Source: CAD feature listing. Evaluate the final solid. Frame: model axes, mm. Round coordinates to 2 decimals unless told otherwise and drop trailing zeros. Loops run counter-clockwise (first coordinate to the right, second up) from the corner with the lowest first, then second, coordinate; pieces in that order, holes last. Notation, with made-up numbers: (-5, 17) -> (28, 17) arc R24 cw to (28, 30) -> close; hole circle Ø3 at (20, 25.5). An arc over 180 degrees is marked (long way). Write item = value, one per line.
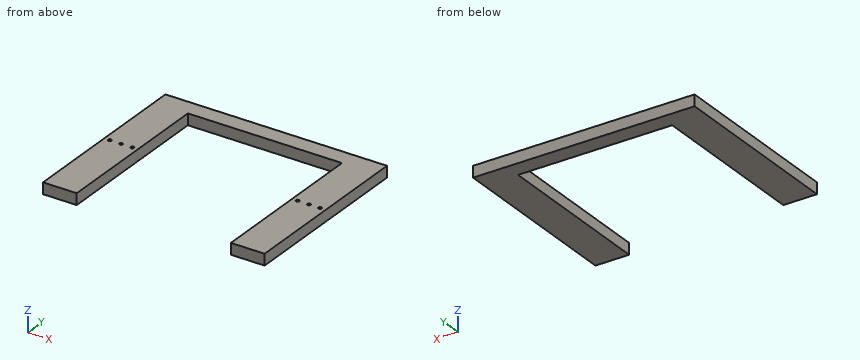
from build123d import *

# Parameters (mm, degrees)
SKETCH_1_W          = 60
SKETCH_1_H          = 325
EXTRUDE_1_DEPTH     = 20
EXTRUDE_1_2_DEPTH   = 20
SKETCH_3_R          = 3
CUT_EXTRUDE_1_DEPTH = 10
SKETCH_5_W          = 274
SKETCH_5_H          = 30
EXTRUDE_2_DEPTH     = 20


with BuildPart() as part:
    # Sketch 1 → Extrude 1 (new body)
    with BuildSketch(Plane.XY):
        with Locations((30, -162.5)):
            Rectangle(SKETCH_1_W, SKETCH_1_H)
    extrude(amount=EXTRUDE_1_DEPTH)


with BuildPart() as body_2:
    # Sketch 1 → Extrude 1 2 (new body)
    with BuildSketch(Plane.XY):
        with Locations((-304, -162.5)):
            Rectangle(SKETCH_1_W, SKETCH_1_H)
    extrude(amount=EXTRUDE_1_2_DEPTH)


with BuildPart() as cut_extrude_1_tool:
    # Sketch 3 → Cut-Extrude 1 (new body)
    with BuildSketch(Plane.XY.offset(20)):
        with Locations((50, -162.5)):
            Circle(SKETCH_3_R)
        with Locations((10, -162.5)):
            Circle(SKETCH_3_R)
        with Locations((30, -162.5)):
            Circle(SKETCH_3_R)
        with Locations((-324, -162.5)):
            Circle(SKETCH_3_R)
        with Locations((-304, -162.5)):
            Circle(SKETCH_3_R)
        with Locations((-284, -162.5)):
            Circle(SKETCH_3_R)
    extrude(amount=-CUT_EXTRUDE_1_DEPTH)


with BuildPart() as part_1:
    add(part.part)

    # Cut-Extrude 1: cut by cut_extrude_1_tool
    add(cut_extrude_1_tool.part, mode=Mode.SUBTRACT)



with BuildPart() as body_2_1:
    add(body_2.part)

    # Cut-Extrude 1: cut by cut_extrude_1_tool
    add(cut_extrude_1_tool.part, mode=Mode.SUBTRACT)


with BuildPart() as part_2:
    add(part_1.part)

    add(body_2_1.part)  # Extrude 2 merges body 2
    # Sketch 5 → Extrude 2 (add)
    with BuildSketch(Plane.XY.offset(20)):
        with Locations((-137, -15)):
            Rectangle(SKETCH_5_W, SKETCH_5_H)
    extrude(amount=-EXTRUDE_2_DEPTH)


solid = part_2.part
1. Section query A-A (y = -144.5). Return the cut outline in (x, z).
Evaluation:
outline = (-334, 0) -> (-274, 0) -> (-274, 20) -> (-334, 20) -> close; (0, 0) -> (60, 0) -> (60, 20) -> (0, 20) -> close
2. Line query: probe 1 along Y at (x, z) = (50, 14.75); probe 2 along X at (y, z) = (-236.5, 3.25); probe 3 along Y at (x, z) = (-177, 13.5). Output: solid intervals per line, ascending. Write a range as from..to.
Evaluation:
probe_1 = -325..-165.5, -159.5..0
probe_2 = -334..-274, 0..60
probe_3 = -30..0
3. Contact query for flat-ended pins moving along their axis: pin 1 Ø1.8 at (x, y) = (49, -163) entering from +Z; pin 2 Ø3 at (x, z) = (-49.5, 13.5) entering from -Y. Output: stop coordinate, or through.
Evaluation:
pin_1 = 10
pin_2 = -30
4. Section query C-C (x = -123.5). Return the cut outline in (y, z), then the cut area to 3 significant figures.
Evaluation:
outline = (-30, 0) -> (0, 0) -> (0, 20) -> (-30, 20) -> close
area = 600 mm²
5. Section query B-B (z = 5.75). Return the cut outline in (x, y), then the cut area to 3 significant figures.
Evaluation:
outline = (-334, -325) -> (-274, -325) -> (-274, -30) -> (0, -30) -> (0, -325) -> (60, -325) -> (60, 0) -> (-334, 0) -> close
area = 47,200 mm²
